The listing builds one solid part. Answer for the finished solid, in the listing's coordinates (mm). A direction names the side the tool comes from. Round coordinates to 2 decimals unless told otherwise and drop trailing zeros. Write each loop counter-clockwise with the first axis right and the second up, starting at its lowest first coordinate (ties: lowest second). Pieces come first, ordered by that corner, then holes. Notation, with made-up numbers: (44, 20) - (69, 20) arc R6 ccw to (69, 26) - close; hole circle Ø1 at (-6.75, -20.5). An arc over 180 degrees is marked (long way). Answer as CSV lines item,"result". Start each with the question number.
Item 1: A cutting plane is placed at B-B on z = -4. Determine the outline of the cut face in (x, y), and give its area (3 significant figures).
Item 2: Flat-ended cylindrical pins translate along their axes: pin 1 (2.5 mm diameter, centred on x = 4, z = -4, fed in from -Y); pin 2 (2 mm diameter, centred on x = 4, z = -5, fed in from -Y); pin 3 (1 mm diameter, centred on x = 4, y = 1, fed in from +Z). Find the tip coordinate at first contact, or state that the pin passes through.
Item 3: For a pull along X with two mould halves and no side action, classify faces 4 (the flat face through (16, -2, -12)), 5 (the cylindrical face through (1.615, 0.74, -4.751)), 6 (the flat face through (4, 1.5, -4)) as pulls with the +X half, pulls with the -X half, needs draft (parallel to the pull), parting line crosses it, or undercut.
Item 4: A cutting plane is placed at C-C on x = 8. Determine the outline of the cut face in (y, z).
Item 5: Straight lines are drawn through the part: line 1 along Z through (x, y) = (4, -0.45); line 2 along X through (y, z) = (-0.35, -4); line 3 along Z through (x, y) = (10.25, -1.5). For each, find the intervals that lie inside material, in ascending order. Write a range as [from, to].
Item 6: A cutting plane is placed at A-A on y = -2.3. Determine the outline of the cut face in (x, z), and give its area (3 significant figures).
Item 7: A cutting plane is placed at D-D on z = -16. Determine the outline of the cut face in (x, y), and give its area (3 significant figures).
Item 8: Which of the six approach directions +Z, -Z, +X, -X, +Y, -Y give full straight-line access (tool end or side, diameter ignored) to faces 1 (the flat face through (15, -2, -12)), 2 (the cylindrical face through (2.85, 0.74, -9.78)), 3 (the flat face through (15.15, -3.2, -11.06))?
Autodesk Inventor part; units mm, degrees
ref_plane "YZ Plane" through (0, 0, 0) normal (1, 0, 0) x (0, 1, 0)
ref_plane "XZ Plane" through (0, 0, 0) normal (0, 1, 0) x (-1, 0, 0)
ref_plane "XY Plane" through (0, 0, 0) normal (0, 0, 1) x (1, 0, 0)
sketch "草圖1" plane through (0, 0, 0) normal (0, 1, 0) x (-1, 0, 0)
  line L0 (0, 0) -> (-16, 0)
  line L1 (-16, 0) -> (-16, -24)
  line L2 (-16, -24) -> (0, -24)
  line L3 (0, -24) -> (0, 0)
  dimension "長" = 16
  dimension "寬" = 24
extrude "樂高擠出" add sketch "草圖1" against normal blind 3.2
sketch "草圖2" plane through (0, 0, 0) normal (0, 1, 0) x (-1, 0, 0)
  circle A0 centre (-12, -4) radius 2.5
  line L0 (-16, 0) -> (-16, -24)
  line L1 (0, 0) -> (-16, 0)
  dimension "d4" = 5
  dimension "d5" = 4
  dimension "d6" = 4
extrude "圓柱擠出" add sketch "草圖2" along normal blind 1.5
pattern_linear "頂部圓柱" count 3 spacing 8 along (0, 0, -1) count 2 spacing 8 along (-1, 0, 0) of "圓柱擠出"
shell "薄殼2" thickness 1 removed faces 1 at (10.666667, -3.2, -16)
sketch "草圖6" plane through (1, -1, -1) normal (0, -1, 0) x (1, 0, 0)
  circle A0 centre (3, -19) radius 1.5
  circle A1 centre (3, -11) radius 1.5
  circle A2 centre (3, -3) radius 1.5
  circle A3 centre (11, -19) radius 1.5
  circle A4 centre (11, -11) radius 1.5
  circle A5 centre (11, -3) radius 1.5
  line L0 (14, 0) -> (14, -22)
  line L1 (0, 0) -> (14, 0)
  line L2 (0, -22) -> (0, 0)
  line L3 (14, -22) -> (0, -22)
  circle A6 centre (7, -7) radius 3.156854
  circle A7 centre (11, -11) radius 2.5
  circle A8 centre (11, -3) radius 2.5
  circle A9 centre (3, -3) radius 2.5
  circle A10 centre (7, -7) radius 2.156854
  point P0 (-1, 1)
  dimension "d41" = 1
extrude "擠出7" add sketch "草圖6" along normal up to surface (2.2 mm away) contours A6
pattern_linear "矩形陣列3" count 2 spacing 8 along (0, 0, -1) of "擠出7"
properties part number "0401_練習"
Geometry says:
1,outline,"(0, -3.2) - (1, -3.2) - (1, -1) - (2.5, -1) - (2.5, 0.5) - (5.5, 0.5) - (5.5, -1) - (10.5, -1) - (10.5, 0.5) - (13.5, 0.5) - (13.5, -1) - (15, -1) - (15, -3.2) - (16, -3.2) - (16, 0) - (14.5, 0) - (14.5, 1.5) - (9.5, 1.5) - (9.5, 0) - (6.5, 0) - (6.5, 1.5) - (1.5, 1.5) - (1.5, 0) - (0, 0) - close"
1,area,"26.4 mm^2"
2,pin 1,"stops at y = 0.5"
2,pin 2,"stops at y = -1"
2,pin 3,"stops at z = -1.5"
3,face 4,"pulls with the +X half"
3,face 5,"undercut"
3,face 6,"needs draft"
4,outline,"(-3.2, -24) - (0, -24) - (0, 0) - (-3.2, 0) - (-3.2, -1) - (-1, -1) - (-1, -4.84) - (-3.2, -4.84) - (-3.2, -5.84) - (-1, -5.84) - (-1, -10.16) - (-3.2, -10.16) - (-3.2, -11.16) - (-1, -11.16) - (-1, -12.84) - (-3.2, -12.84) - (-3.2, -13.84) - (-1, -13.84) - (-1, -18.16) - (-3.2, -18.16) - (-3.2, -19.16) - (-1, -19.16) - (-1, -23) - (-3.2, -23) - close"
5,line 1,"z = [-24, -21.5], [-18.5, -13.5], [-10.5, -5.5], [-2.5, 0]"
5,line 2,"x = [0, 2.5], [5.5, 10.5], [13.5, 16]"
5,line 3,"z = [-24, -23], [-18.21, -13.79], [-10.21, -5.79], [-1, 0]"
6,outline,"(0, -24) - (16, -24) - (16, 0) - (0, 0) - close; circle Ø6.31 at (8, -16); circle Ø6.31 at (8, -8); hole (1, -23) - (15, -23) - (15, -1) - (1, -1) - close; hole circle Ø4.31 at (8, -16); hole circle Ø4.31 at (8, -8)"
6,area,"109 mm^2"
7,outline,"(0, -3.2) - (1, -3.2) - (1, -1) - (4.84, -1) - (4.84, -3.2) - (5.84, -3.2) - (5.84, -1) - (10.16, -1) - (10.16, -3.2) - (11.16, -3.2) - (11.16, -1) - (15, -1) - (15, -3.2) - (16, -3.2) - (16, 0) - (0, 0) - close"
7,area,"24.8 mm^2"
8,face 1,"-Y"
8,face 2,"+Y"
8,face 3,"+Z, -Z, +X, -X, -Y"
